Could you check a few things on this drawing? It's one solid part, dimensions in mm from its lowest x, y, z. Coordinates: 2 decimals unless noted, no trailing zeros. Write each loop counter-clockwise with the first axis right and the second up, starting at its lowest first coordinate (ties: lowest second). Pieces come first, ordered by that corner, then holes. Notation, with made-up numbers: M 34,42.5 L 49,42.5 A28 cw 49,80.5 Z; hole C 20.25,-2.5 d4. An arc over 180 degrees is marked long. Use a Markdown table: item, result.
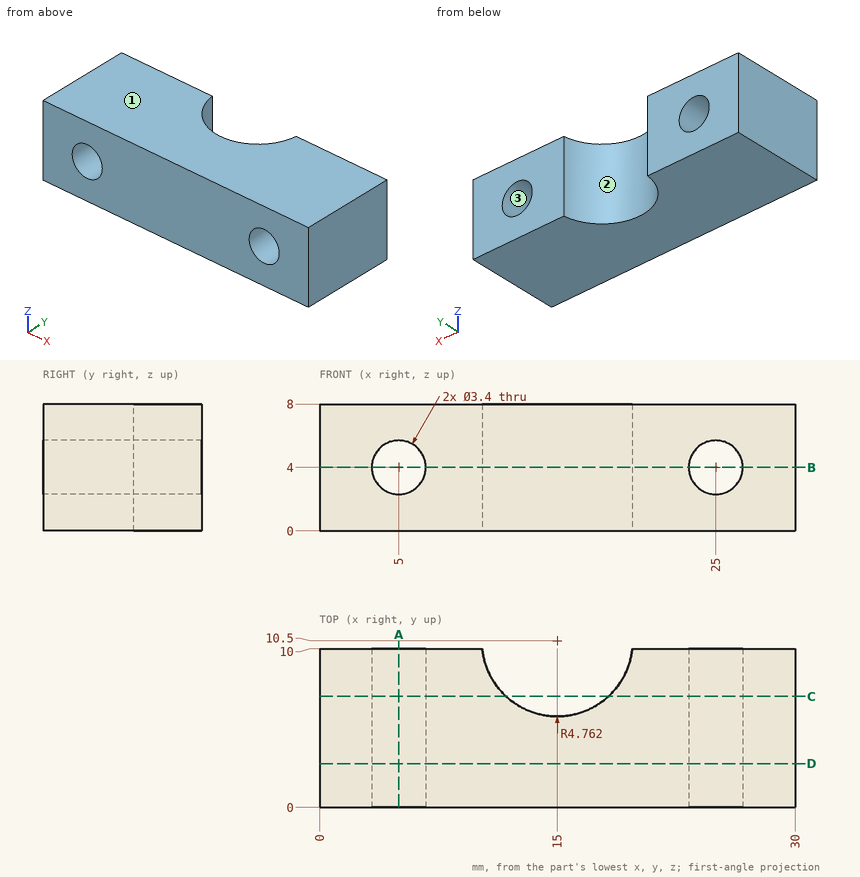
1. Suppose I cut it at B-B on z = 4. Write out the boundary of the cut face in (x, y) (1 decimal), and give its area (3 significant figures).
Answers follow:
| item | result |
|---|---|
| outline | M 0,0 L 3.3,0 L 3.3,10 L 0,10 Z; M 6.7,0 L 23.3,0 L 23.3,10 L 19.7,10 A4.8 cw 10.3,10 L 6.7,10 Z; M 26.7,0 L 30,0 L 30,10 L 26.7,10 Z |
| area | 201 mm2 |
2. Suppose I cut it at C-C on y = 7. Write out the boundary of the cut face in (x, z).
Answers follow:
| item | result |
|---|---|
| outline | M 0,0 L 11.77,0 L 11.77,8 L 0,8 Z; M 18.23,0 L 30,0 L 30,8 L 18.23,8 Z; hole C 5,4 d3.4; hole C 25,4 d3.4 |
3. Will this pin go through, and if not, where does the flat tip stop? pin 1 Ø3 at (x, z) = (25, 4) entering from -Y.
Answers follow:
| item | result |
|---|---|
| pin 1 | passes through |
4. Suppose I cut it at D-D on y = 2.75. Write out the boundary of the cut face in (x, z).
Answers follow:
| item | result |
|---|---|
| outline | M 0,0 L 30,0 L 30,8 L 0,8 Z; hole C 5,4 d3.4; hole C 25,4 d3.4 |
5. I need wall thicknesses on probe 1 along Z at (x, y) = (25, 6.5); probe 2 along X at (y, z) = (3, 4.5) (1 decimal); probe 3 along Z at (x, y) = (6, 4.25) (1 decimal). Which ranges of each line are inside material? Lowest first, please.
Answers follow:
| item | result |
|---|---|
| probe 1 | z = 0 to 2.3, 5.7 to 8 |
| probe 2 | x = 0 to 3.4, 6.6 to 23.4, 26.6 to 30 |
| probe 3 | z = 0 to 2.6, 5.4 to 8 |
6. Suppose I cut it at A-A on x = 5. Write out the boundary of the cut face in (y, z).
Answers follow:
| item | result |
|---|---|
| outline | M 0,0 L 10,0 L 10,2.3 L 0,2.3 Z; M 0,5.7 L 10,5.7 L 10,8 L 0,8 Z |
7. We'd pull the mould along Z, two halves only. Please class the marked faces 1, 2 and 3: +Z half, -Z half, draft (parallel to the pull), parting line (faces both ways), or undercut.
Answers follow:
| item | result |
|---|---|
| face 1 | +Z half |
| face 2 | draft |
| face 3 | undercut |
